Geometry check sheet. Reference: the model listing, model coordinates, mm. A direction names the side the tool comes from. Give positions to 0.01 mm unless a question says otherwise; leave off trailing zeros. Write each loop counter-clockwise with the first axis right and the second up, starting at its lowest first coordinate (ties: lowest second). Pieces come first, ordered by that corner, then holes. Notation, with made-up numbers: (55, 0.5) - (93, 0.5) arc R16 cw to (93, 29.5) - close; hole circle Ø8 at (34, 42.5). An arc over 180 degrees is marked (long way). One line per question, with ' | ' between items. Start each with the question number.
Q1. Release check for a two-part mould opening along Y. For faces 1 (the face through (-4.95, 4.15, -21.38)), 2 (the face through (-8.075, 2.958, -25.759)), 3 (the face through (-0.21, 8.12, 21.77)) record: +Y half, -Y half, draft (parallel to the pull), parting line (faces both ways), or undercut.
Q2. Thickness scan on L1, parallel to X at y = 5, z = 28; L2, parallel to X at y = 4.5, z = -20.5; L3, parallel to Y at x = 5, z = 26. Record the ranges inside material, lowest first. Write a range as [from, to].
Q3. Section check B-B on x = -10.5. Record the boundary of the cut face in (y, z).
Q4. Set-up check for faces 4 (the face through (-4.73, 3.78, 25.64)), 5 (the face through (5, 6, -18)), 6 (the face through (-8.5, 3, -20.7)), 7 (the face through (-1.5, 3, -24.5)), 8 (the face through (-2.145, 2.958, -18.654)): record each of +Z, -Z, +X, -X, +Y, -Y from which the full face is reachable in a straight line by a thin tool's end or side.
Q5. Gauge pin test, flat ends, axial feed: P1, Ø3, axis at y = 3, z = 21.5, coming from the -X side; P2, Ø1.4, axis at y = 1.5, z = -22.5, coming from the -X side; P3, Ø1.5, axis at x = -3, z = -20, coming from the +Y side. Record the tip position at first contact, or that the pin passes through.
Q6. Section check C-C on z = 10.5. Record the boundary of the cut face in (x, y).
Q7. Section check A-A on z = 0. Record the boundary of the cut face in (x, y), and give its area (3 significant figures).
Q8. Section check D-D on z = 22.5. Record the boundary of the cut face in (x, y).
```python
from build123d import *

# Parameters (mm, degrees)
SKETCH_1_R            = 18
EXTRUDE_1_DEPTH       = 6
SKETCH_4_W            = 3
SKETCH_4_H            = 5
CUT_EXTRUDE_2_DEPTH   = 6
SKETCH_20_W           = 30
SKETCH_20_H           = 10
EXTRUDE_6_DEPTH       = 4
EXTRUDE_5_DEPTH       = 6
HOLE_WIZARD_M32_D     = 3.4
HOLE_WIZARD_M32_DEPTH = 7
M3X0_51_D             = 2.5
M3X0_52_D             = 2.5
M3X0_52_DEPTH         = 8.5
M3X0_52_TIP           = 0.751075774
FILLET_1_R            = 2
FILLET_2_R            = 3
CHAMFER_1_SIZE        = 3.7


with BuildPart() as part:
    # Эскиз1 → Бобышка-Вытянуть1 (new body)
    with BuildSketch(Plane(origin=(0, 0, 0), x_dir=(1, 0, 0), z_dir=(0, 1, 0))):
        with BuildLine():
            Line((-15, -14.696938457), (-15, -29.949874371))
            Line((-15, -29.949874371), (15, -29.949874371))
            Line((15, -29.949874371), (15, -14.696938457))
            ThreePointArc((15, -14.696938457), (0, 21), (-15, -14.696938457))
        make_face()
        with Locations(Location((0, 0, 0), (0, 0, 270))):
            Circle(SKETCH_1_R, mode=Mode.SUBTRACT)
    extrude(amount=EXTRUDE_1_DEPTH)

    # Эскиз4 → Вырез-Вытянуть2 (cut)
    with BuildSketch(Plane(origin=(0, 6, 0), x_dir=(1, 0, 0), z_dir=(0, 1, 0))):
        with Locations((0, 18.5)):
            Rectangle(SKETCH_4_W, SKETCH_4_H)
    extrude(amount=-CUT_EXTRUDE_2_DEPTH, mode=Mode.SUBTRACT)

    # Эскиз20 → Бобышка-Вытянуть6 (add)
    with BuildSketch(Plane(origin=(0, 6, 0), x_dir=(1, 0, 0), z_dir=(0, 1, 0))):
        with Locations((0, -24.949874371)):
            Rectangle(SKETCH_20_W, SKETCH_20_H)
    extrude(amount=EXTRUDE_6_DEPTH)

    # Эскиз11 → Бобышка-Вытянуть5 (add)
    with BuildSketch(Plane(origin=(0, 6, 0), x_dir=(1, 0, 0), z_dir=(0, 1, 0))):
        Polygon((-1.5, 17.937391115), (-8.5, 17.937391115), (-8.5, 26.061746768), (-1.5, 27.937391115), align=None)
        Polygon((8.5, 17.937391115), (8.5, 26.061746768), (1.5, 27.937391115), (1.5, 17.937391115), align=None)
    extrude(amount=-EXTRUDE_5_DEPTH)

    # Отверстие с зазором M32
    with Locations(Plane.ZY.offset(8.5)):
        with Locations((-22.632305569, 3)):
            Hole(HOLE_WIZARD_M32_D / 2, depth=HOLE_WIZARD_M32_DEPTH)

    # Отверстие обработанное метчиком M3x0.51 (through all)
    with Locations(Plane(origin=(1.5, -0.91070238, -4.39340032), x_dir=(0, 0, 1), z_dir=(-1, 0, 0))):
        with Locations((-18.238905249, 3.91070238)):
            Hole(M3X0_51_D / 2)

    # Отверстие обработанное метчиком M3x0.52
    with Locations(Plane.XY.offset(29.949874371)):
        with Locations((-5, 5), (5, 5)):
            Hole(M3X0_52_D / 2, depth=M3X0_52_DEPTH)
            with Locations((0, 0, -(M3X0_52_DEPTH + M3X0_52_TIP / 2))):  # 118° drill point
                Cone(0, M3X0_52_D / 2, M3X0_52_TIP, mode=Mode.SUBTRACT)

    # Скругление1
    fillet_1_edges = [part.edges().sort_by_distance(p)[0] for p in [
        (15, 3, 14.696938457),
        (-8.5, 3, -19.20286437),
        (8.5, 3, -19.20286437),
        (15, 5, 29.949874371),
        (-15, 5, 29.949874371),
        (-15, 3, 14.696938457),
        (8.5, 3, -26.061746768),
        (1.5, 3, -27.937391115),
        (-1.5, 3, -27.937391115),
        (-8.5, 3, -26.061746768),
    ]]
    fillet(fillet_1_edges, radius=FILLET_1_R)

    # Скругление2
    fillet_2_edges = [part.edges().sort_by_distance(p)[0] for p in [
        (-1.5, 3, -17.937391115),
        (1.5, 3, -17.937391115),
    ]]
    fillet(fillet_2_edges, radius=FILLET_2_R)

    # Фаска1
    chamfer_1_edges = [part.edges().sort_by_distance(p)[0] for p in [
        (0, 10, 19.949874371),
    ]]
    chamfer(chamfer_1_edges, length=CHAMFER_1_SIZE)


solid = part.part
```
Working result:
1) face 1: undercut | face 2: draft | face 3: +Y half
2) L1: x = [-15, -6.25], [-3.75, 3.75], [6.25, 15] | L2: x = [-8.5, -1.5], [1.5, 8.5] | L3: y = [0, 3.75], [6.25, 10]
3) outline: (0, -18.19) - (6, -18.19) - (6, -14.62) - (0, -14.62) - close; (0, 14.62) - (6, 14.62) - (6, 19.95) - (6.3, 19.95) - (10, 23.65) - (10, 29.95) - (0, 29.95) - close
4) face 4: +Z | face 5: -Z, +X, -X, +Y | face 6: -Z, -X, +Y, -Y | face 7: -Z, +Y, -Y | face 8: +Y, -Y
5) P1: stops at x = -15 | P2: stops at x = -8.5 | P3: stops at y = 6
6) outline: (-18.19, 0) - (-14.62, 0) - (-14.62, 6) - (-18.19, 6) - close; (14.62, 0) - (18.19, 0) - (18.19, 6) - (14.62, 6) - close
7) outline: (-21, 0) - (-18, 0) - (-18, 6) - (-21, 6) - close; (18, 0) - (21, 0) - (21, 6) - (18, 6) - close | area: 36.0 mm2
8) outline: (-15, 0) - (15, 0) - (15, 8.85) - (-15, 8.85) - close; hole circle Ø2.5 at (-5, 5); hole circle Ø2.5 at (5, 5)
